Design review of the part built by this model. Coordinates are the model's own, in mm. A direction names the side the tool comes from. Coordinates: 2 decimals unless noted, no trailing zeros. Write each loop counter-clockwise with the first axis right and the second up, starting at its lowest first coordinate (ties: lowest second). Pieces come first, ordered by that corner, then holes. Notation, with made-up numbers: (82, 74) - (90, 74) arc R7 cw to (90, 82) - close; hole circle Ø1 at (-15.5, -17.5). An arc over 180 degrees is marked (long way). Use a Markdown table: item, result.
from build123d import *

# Parameters (mm, degrees)
SKETCH1_W           = 35
SKETCH1_H           = 25
SKETCH1_R           = 0.75
SKETCH1_R_2         = 2.5
BOSS_EXTRUDE1_DEPTH = 5
SKETCH5_R           = 1.5
BOSS_EXTRUDE3_DEPTH = 12
SKETCH4_W           = 25
SKETCH4_H           = 40
BOSS_EXTRUDE2_DEPTH = 5
CUT_EXTRUDE2_REACH  = 55.819
SKETCH3_R           = 1.5
SKETCH3_W           = 13.2
SKETCH3_H           = 23.5
FILLET5_R           = 1.5
FILLET6_R           = 2


with BuildPart() as part:
    # Sketch1 → Boss-Extrude1 (new body)
    with BuildSketch(Plane(origin=(0, 0, 0), x_dir=(0, 0, -1), z_dir=(1, 0, 0))):
        Rectangle(SKETCH1_W, SKETCH1_H)
        with Locations((-14.45, 0)):
            Circle(SKETCH1_R, mode=Mode.SUBTRACT)
        with Locations((-12.45, 0)):
            Circle(SKETCH1_R, mode=Mode.SUBTRACT)
        with Locations((-10.45, 0)):
            Circle(SKETCH1_R, mode=Mode.SUBTRACT)
        with Locations((-8.45, 0)):
            Circle(SKETCH1_R, mode=Mode.SUBTRACT)
        with Locations((-6.45, 0)):
            Circle(SKETCH1_R, mode=Mode.SUBTRACT)
        with Locations((-4.45, 0)):
            Circle(SKETCH1_R, mode=Mode.SUBTRACT)
        with Locations((4.45, 0)):
            Circle(SKETCH1_R, mode=Mode.SUBTRACT)
        with Locations((6.45, 0)):
            Circle(SKETCH1_R, mode=Mode.SUBTRACT)
        with Locations((8.45, 0)):
            Circle(SKETCH1_R, mode=Mode.SUBTRACT)
        with Locations((10.45, 0)):
            Circle(SKETCH1_R, mode=Mode.SUBTRACT)
        with Locations((12.45, 0)):
            Circle(SKETCH1_R, mode=Mode.SUBTRACT)
        with Locations((14.45, 0)):
            Circle(SKETCH1_R, mode=Mode.SUBTRACT)
        Circle(SKETCH1_R_2, mode=Mode.SUBTRACT)
    extrude(amount=BOSS_EXTRUDE1_DEPTH)

    # Sketch5 → Boss-Extrude3 (add)
    with BuildSketch(Plane(origin=(5, 0, 0), x_dir=(0, 0, -1), z_dir=(1, 0, 0))):
        with Locations((-14.5, 9.5)):
            Circle(SKETCH5_R)
        with Locations((14.5, 9.5)):
            Circle(SKETCH5_R)
        with Locations((14.5, -9.5)):
            Circle(SKETCH5_R)
        with Locations((-14.5, -9.5)):
            Circle(SKETCH5_R)
    extrude(amount=BOSS_EXTRUDE3_DEPTH)

    # Sketch4 → Boss-Extrude2 (add)
    with BuildSketch(Plane(origin=(17, 17.5, 0), x_dir=(0, -1, 0), z_dir=(1, 0, 0))):
        with Locations((17.5, 2.5)):
            Rectangle(SKETCH4_W, SKETCH4_H)
    extrude(amount=BOSS_EXTRUDE2_DEPTH)

    # Sketch3 → Cut-Extrude2 (cut, up to next)
    with BuildSketch(Plane(origin=(22, 0, -30), x_dir=(0, 1, 0), z_dir=(1, 0, 0)), mode=Mode.PRIVATE) as cut_extrude2_sk1:
        with Locations(Location((0, 38.75, 0), (0, 0, 270))):
            Circle(SKETCH3_R)
    cut_extrude2_tool1 = extrude(cut_extrude2_sk1.sketch, amount=-CUT_EXTRUDE2_REACH, mode=Mode.PRIVATE) & part.part
    # Sketch3 → Cut-Extrude2 (cut, up to next)
    with BuildSketch(Plane(origin=(22, 0, -30), x_dir=(0, 1, 0), z_dir=(1, 0, 0)), mode=Mode.PRIVATE) as cut_extrude2_sk2:
        with Locations(Location((0, 10.95, 0), (0, 0, 270))):
            Circle(SKETCH3_R)
    cut_extrude2_tool2 = extrude(cut_extrude2_sk2.sketch, amount=-CUT_EXTRUDE2_REACH, mode=Mode.PRIVATE) & part.part
    # Sketch3 → Cut-Extrude2 (cut, up to next)
    with BuildSketch(Plane(origin=(22, 0, -30), x_dir=(0, 1, 0), z_dir=(1, 0, 0)), mode=Mode.PRIVATE) as cut_extrude2_sk3:
        with Locations((0, 24.85)):
            Rectangle(SKETCH3_W, SKETCH3_H)
    cut_extrude2_tool3 = extrude(cut_extrude2_sk3.sketch, amount=-CUT_EXTRUDE2_REACH, mode=Mode.PRIVATE) & part.part
    add(cut_extrude2_tool1.solids().sort_by_distance((22, 0, 8.75))[0], mode=Mode.SUBTRACT)
    add(cut_extrude2_tool2.solids().sort_by_distance((22, 0, -19.05))[0], mode=Mode.SUBTRACT)
    add(cut_extrude2_tool3.solids().sort_by_distance((22, 0, -5.15))[0], mode=Mode.SUBTRACT)

    # Fillet5
    fillet5_edges = [part.edges().sort_by_distance(p)[0] for p in [
        (19.5, 6.6, 6.6),
        (19.5, -6.6, 6.6),
        (19.5, -6.6, -16.9),
        (19.5, 6.6, -16.9),
    ]]
    fillet(fillet5_edges, radius=FILLET5_R)

    # Fillet6
    fillet6_edges = [part.edges().sort_by_distance(p)[0] for p in [
        (2.5, 12.5, 17.5),
        (2.5, 12.5, -17.5),
        (2.5, -12.5, -17.5),
        (2.5, -12.5, 17.5),
        (19.5, 12.5, -22.5),
        (19.5, 12.5, 17.5),
        (19.5, -12.5, 17.5),
        (19.5, -12.5, -22.5),
    ]]
    fillet(fillet6_edges, radius=FILLET6_R)


solid = part.part
(1) Take a section at C-C on x = 19.5. Write out the cut boundary in (y, z).
Determined:
| item | result |
|---|---|
| outline | (-12.5, -20.5) arc R2 ccw to (-10.5, -22.5) - (10.5, -22.5) arc R2 ccw to (12.5, -20.5) - (12.5, 15.5) arc R2 ccw to (10.5, 17.5) - (-10.5, 17.5) arc R2 ccw to (-12.5, 15.5) - close; hole (-6.6, -15.4) arc R1.5 ccw to (-5.1, -16.9) - (5.1, -16.9) arc R1.5 ccw to (6.6, -15.4) - (6.6, 5.1) arc R1.5 ccw to (5.1, 6.6) - (-5.1, 6.6) arc R1.5 ccw to (-6.6, 5.1) - close; hole circle Ø3 at (0, -19.05); hole circle Ø3 at (0, 8.75) |
(2) Take a section at A-A on z = -19.05. Write out the cut boundary in (x, y).
Determined:
| item | result |
|---|---|
| outline | (17, -12.5) - (22, -12.5) - (22, -1.5) - (17, -1.5) - close; (17, 1.5) - (22, 1.5) - (22, 12.5) - (17, 12.5) - close |
(3) Machinability: for faces 1 (the cylindrical face through (2.5, 0, 9.2)), 2 (the cylindrical face through (10.9, -10.4, 15.7)), 3 (the cylindrical face through (19.46, -6.17, -16.45)), 4 (the cylindrical face through (2.54, -11.93, -16.9)), 5 (the cylindrical face through (2.5, 0, 13.2)), which of the approach directions +Z, -Z, +X, -X, +Y, -Y give a long, thin tool a straight path to every point of the face, cutting with its end or side? Answer none if there is none.
Determined:
| item | result |
|---|---|
| face 1 | +X, -X |
| face 2 | none |
| face 3 | +X |
| face 4 | -Z, -X, -Y |
| face 5 | -X |
(4) Draft analysis for pull direction Z (two halves, no side actions). For faces 6 (the flat face through (19, 12.5, -2)), 7 (the cylindrical face through (2.5, 0, 15.2)), 8 (the cylindrical face through (19.54, -11.9, 16.93)), state which applies: +Z half, -Z half, draft (parallel to the pull), parting line (faces both ways), or undercut.
Determined:
| item | result |
|---|---|
| face 6 | draft |
| face 7 | undercut |
| face 8 | +Z half |
(5) For pin 1 (5.5 mm diameter, centred on x = 1.5, y = 0, fed in from -Z); pin 2 (1.7 mm diameter, centred on y = 0, z = -10.45, fed in from +X); pin 3 (1.5 mm diameter, centred on x = 16, y = -8, fed in from -Z), all flat-tipped, find the tip position at first contact; note any pin that passes through.
Determined:
| item | result |
|---|---|
| pin 1 | z = -17.5 |
| pin 2 | x = 5 |
| pin 3 | z = -15.8 |
(6) Take a section at D-D on y = -9.5. Write out the cut boundary in (x, z).
Determined:
| item | result |
|---|---|
| outline | (0, -17.5) - (5, -17.5) - (5, -16) - (17, -16) - (17, -22.5) - (22, -22.5) - (22, 17.5) - (17, 17.5) - (17, 16) - (5, 16) - (5, 17.5) - (0, 17.5) - close; hole (5, -13) - (17, -13) - (17, 13) - (5, 13) - close |
(7) Take a section at B-B on z = 12.45. Write out the cut boundary in (x, y), and give its area (4 significant figures).
Determined:
| item | result |
|---|---|
| outline | (0, -12.5) - (5, -12.5) - (5, -0.75) - (0, -0.75) - close; (0, 0.75) - (5, 0.75) - (5, 12.5) - (0, 12.5) - close; (17, -12.5) - (22, -12.5) - (22, 12.5) - (17, 12.5) - close |
| area | 242.5 mm2 |
(8) For L1, parallel to X at y = 5.75, z = 10; L2, parallel to Y at x = 2.8, z = -14.45; L3, parallel to Y at x = 20.25, z = 1, list the stretches that pass through material, from the lowest coordinate up. Write a range as from..to.
Determined:
| item | result |
|---|---|
| L1 | 0..5, 17..22 |
| L2 | -12.5..-0.75, 0.75..12.5 |
| L3 | -12.5..-6.6, 6.6..12.5 |
